```python
from build123d import *
from build123d import SkipClean  # not in build123d's __all__

# Parameters (mm, degrees)
F1_ANGLE = 90
F2_R     = 6.35
F3_DEPTH = 101.6
F5_DEPTH = 6.35


with BuildPart() as f1:
    # F0 (on Front) → F1 (revolve)
    with BuildSketch(Plane.XZ):
        Polygon((0, -10.9985226281), (0, 0), (-6.35, 0), align=None)
    revolve(axis=Axis((0, 0, -5.499261314), (0, 0, -1)), revolution_arc=F1_ANGLE)

    # F2 (on face) → F3 (join)
    with BuildSketch(Plane.XY):
        Circle(F2_R)
    extrude(amount=F3_DEPTH)

    # F4 (on face) → F5 (join)
    with BuildSketch(Plane.XY.offset(101.6)):
        with BuildLine():
            ThreePointArc((0, -6.35), (4.4901280605, -4.4901280605), (6.35, 0))
            Line((6.35, 0), (0, 0))
            Line((0, 0), (0, -6.35))
        make_face()
    with SkipClean():  # cleaning this boolean's faces spoils the solid; the shape is the same uncleaned
        extrude(amount=F5_DEPTH)


solid = f1.part
```
Work out the finished part from the listing and answer in its coordinate system (mm). A direction names the side the tool comes from. Give positions to 0.01 mm unless a question says otherwise; leave off trailing zeros. Order: outer loops, then holes, each group sorted by start corner. A loop starts at its lowest first (then second) coordinate and runs counter-clockwise, first axis right, second up.
1. Section A-A, the plane x = 1.75 is taken. Determine the outline of the cut face in (y, z).
Result sheet:
outline: (-6.1, 0) - (6.1, 0) - (6.1, 101.6) - (0, 101.6) - (0, 107.95) - (-6.1, 107.95) - close
2. Each of these flat-tipped pins is pushed along its axis until it touches: P1, Ø2, axis at y = 2.5, z = 56.5, coming from the +X side; P2, Ø6.5, axis at x = 0, y = 1.5, coming from the +Z side; P3, Ø3, axis at x = -2, z = -8, coming from the -Y side; P4, Ø1, axis at x = 5, y = 1.5, coming from the +Z side. Where does it stop, or does it pass through?
Result sheet:
P1: stops at x = 6.17
P2: stops at z = 107.95
P3: stops at y = 0
P4: stops at z = 101.6
3. Section B-B, the plane z = 16.5 is taken. Determine the outline of the cut face in (x, y).
Result sheet:
outline: circle Ø12.7 at (0, 0)
4. Straight lines are drawn through the part: L1, parallel to Z at x = -5, y = -3; L2, parallel to Z at x = 2, y = -1.25; L3, parallel to Y at x = -0.5, z = 28. For each, find the intervals that lie inside material, in ascending order.
Result sheet:
L1: z = 0 to 101.6
L2: z = 0 to 107.95
L3: y = -6.33 to 6.33
5. For faces 1 (the conical face through (-2.238, 2.189, -5.576)), 2 (the flat face through (3, 0, 105)), 3 (the flat face through (0, -3, 105)), 4 (the flat face through (-2, 0, -3)), 5 (the flat face through (0, 2, -3)), determine the directions among +Z, -Z, +X, -X, +Y, -Y from which every point of the face is accessible in a straight line to the end or side of a thin tool.
Result sheet:
face 1: -Z, -X, +Y
face 2: +Z, +X, -X, +Y
face 3: +Z, -X, +Y, -Y
face 4: -Z, +X, -X, -Y
face 5: -Z, +X, +Y, -Y
